Part model, mm, in its own coordinate system. A direction names the side the tool comes from. Coordinates: 2 decimals unless noted, no trailing zeros. Write each loop counter-clockwise with the first axis right and the second up, starting at its lowest first coordinate (ties: lowest second). Pieces come first, ordered by that corner, then holes. Notation, with made-up numbers: (45.25, 9) -> (93.25, 9) arc R15 cw to (93.25, 22) -> close; hole circle Ø1 at (-15.5, 77.25). An arc over 180 degrees is marked (long way). Write item = value, one per line. Start each with the question number.
Q1. Tool access for faces 1 (the flat face through (101.5, -98, 52)), 2 (the flat face through (64, -100, 39)): list every direction of +Z, -Z, +X, -X, +Y, -Y with a clear straight run to the whole face (end or side of a thin tool).
Q2. Probe line 1 (Z direction, x = 67.5, y = -98.6); line 2 (Z direction, x = 110, y = -97.7); line 3 (X direction, y = -97.4, z = 57). List the from-to ranges inside material, lowest first.
Q3. Band-saw the part on B-B, the plane z = 50. List the corners of the cut face in (x, y).
Q4. Band-saw the part on A-A, the plane x = 34. List the corners of the cut face in (y, z), plus the area to 3 significant figures.
Q5. Pin check, flat tip, straight feed: P1, Ø1.2, axis at x = 83.5, y = -97.5, coming from the -Z side. Stop position of the tip, or through.
Q6. Pull direction X, two halves, no side cores. Call faces 3 (the flat face through (0, -98, 37)), 4 (the flat face through (65, -98, 40)), 5 (the flat face through (130, -98, 37)), 6 (the flat face through (30, -98, 52)): released by +X, released by -X, zero draft, split by the parting line, or undercut.
Q7. Band-saw the part on C-C, the plane y = -98.8. List the corners of the cut face in (x, z), plus the area to 3 significant figures.
from build123d import *

# Parameters (mm, degrees)
SKETCH005_W     = 130
SKETCH005_H     = 76
PAD003_DEPTH    = 4
SKETCH006_W     = 71.5
SKETCH006_H     = 25
POCKET001_DEPTH = 4.001
SKETCH007_R     = 3.6
HOLE001_DEPTH   = 4.001


with BuildPart() as part:
    # Sketch005 → Pad003 (new body)
    with BuildSketch(Plane.XZ.offset(96)):
        with Locations((65, 38)):
            Rectangle(SKETCH005_W, SKETCH005_H)
    extrude(amount=PAD003_DEPTH)

    # Sketch006 (on Face6 of Pad003) → Pocket001 (cut, through all)
    with BuildSketch(Plane.XZ.offset(100)):
        with Locations((65.75, 52.5)):
            Rectangle(SKETCH006_W, SKETCH006_H)
    extrude(amount=-POCKET001_DEPTH, mode=Mode.SUBTRACT)

    # Sketch007 (on Face5 of Pocket001) → Hole001 (cut, through all)
    with BuildSketch(Plane.XZ.offset(100)):
        with Locations((110, 15)):
            Circle(SKETCH007_R)
    extrude(amount=-HOLE001_DEPTH, mode=Mode.SUBTRACT)


solid = part.part
Ans:
q1.face_1 = +Y, -Y
q1.face_2 = +Z, -Z, +X, -X, -Y
q2.line_1 = 0 to 40, 65 to 76
q2.line_2 = 0 to 11.4, 18.6 to 76
q2.line_3 = 0 to 30, 101.5 to 130
q3.outline = (0, -100) -> (30, -100) -> (30, -96) -> (0, -96) -> close; (101.5, -100) -> (130, -100) -> (130, -96) -> (101.5, -96) -> close
q4.outline = (-100, 0) -> (-96, 0) -> (-96, 40) -> (-100, 40) -> close; (-100, 65) -> (-96, 65) -> (-96, 76) -> (-100, 76) -> close
q4.area = 204 mm2
q5.P1 = 0
q6.face_3 = released by -X
q6.face_4 = undercut
q6.face_5 = released by +X
q6.face_6 = undercut
q7.outline = (0, 0) -> (130, 0) -> (130, 76) -> (0, 76) -> close; hole (30, 40) -> (101.5, 40) -> (101.5, 65) -> (30, 65) -> close; hole circle Ø7.2 at (110, 15)
q7.area = 8,050 mm2
